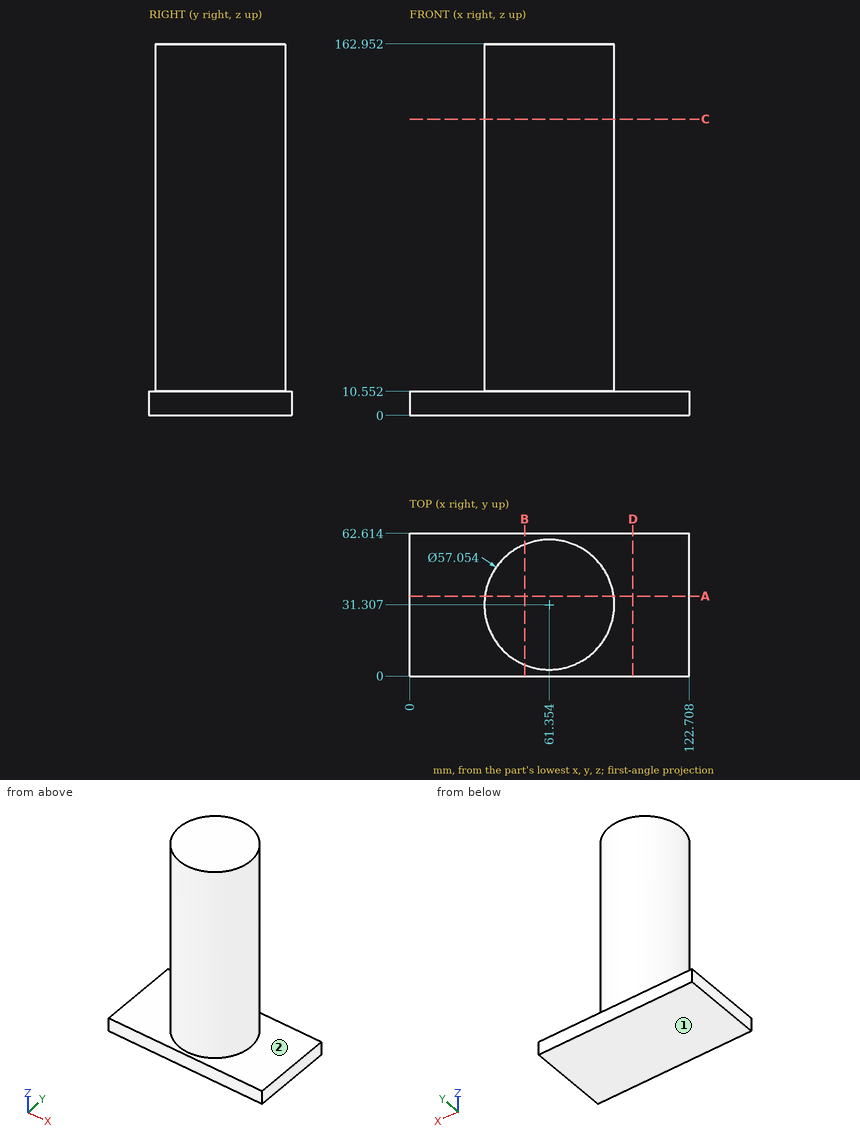
Geometry: see drawing. Coordinates: mm, zero at the bounding-box minimum. A direction names the side the tool comes from. Coordinates: 2 decimals unless noted, no trailing zeros. Loops run counter-clockwise (first coordinate to the right, second up) from the corner with the lowest first, then second, coordinate; pieces in that order, holes last. Notation, with made-up numbers: (32, -13) - (56, -13) arc R11 ccw to (56, 3) - close; hole circle Ø10 at (55.5, 5.5). An arc over 180 degrees is marked (long way). Answer as CSV lines item,"result".
1. Contact query for flat-ended pins moving along their axis: pin 1 (3 mm diameter, centred on y = 32.5, z = 94, fed in from -X); pin 2 (5 mm diameter, centred on y = 43, z = 87, fed in from +X); pin 3 (1.5 mm diameter, centred on y = 44.5, z = 101, fed in from +X). Output: stop coordinate, or through.
Established:
pin 1,"stops at x = 32.83"
pin 2,"stops at x = 88.36"
pin 3,"stops at x = 87.02"
2. Section C-C (z = 130). Return loops of the section in (x, y).
Established:
outline,"circle Ø57.05 at (61.35, 31.31)"
3. Ray query, line 1 (Z direction, x = 28, y = 22); line 2 (X direction, y = 26, z = 115.5) (1 decimal); line 3 (Y direction, x = 87.5, z = 98.5) (1 decimal). Return the intervals inside material, ascending.
Established:
line 1,"z = 0 to 10.55"
line 2,"x = 33.3 to 89.4"
line 3,"y = 19.9 to 42.7"
4. Section B-B (x = 50.5). Return loops of the section in (y, z) (1 decimal).
Established:
outline,"(0, 0) - (62.6, 0) - (62.6, 10.6) - (57.7, 10.6) - (57.7, 163) - (4.9, 163) - (4.9, 10.6) - (0, 10.6) - close"
5. Section A-A (y = 35). Return loops of the section in (x, z), then the cut area to 3 significant figures.
Established:
outline,"(0, 0) - (122.71, 0) - (122.71, 10.55) - (89.64, 10.55) - (89.64, 162.95) - (33.07, 162.95) - (33.07, 10.55) - (0, 10.55) - close"
area,"9,920 mm2"
6. Reachability of the marked faces 1 and 2 from +Z, -Z, +X, -X, +Y, -Y: full face, straight path, thin tool, end or side. Return the list, or none.
Established:
face 1,"-Z, +X, -X, +Y, -Y"
face 2,"+Z"
7. Section D-D (x = 98). Return loops of the section in (y, z), then the cut area to 3 significant figures.
Established:
outline,"(0, 0) - (62.61, 0) - (62.61, 10.55) - (0, 10.55) - close"
area,"661 mm2"
